```python
from build123d import *

# Parameters (mm, degrees)
ESQUISSE1_W        = 90
ESQUISSE1_H        = 10
BOSS_EXTRU_1_DEPTH = 10
CHANFREIN1_SIZE    = 20


with BuildPart() as part:
    # Esquisse1 → Boss.-Extru.1 (new body)
    with BuildSketch(Plane.XY):
        Polygon((0, 220), (536, 220), (536, 0), (436, 0), (200, 0), (180, 0), (180, 60), (80, 60), (80, 0), (0, 0), align=None)
        with Locations((118, 175)):
            Rectangle(ESQUISSE1_W, ESQUISSE1_H, mode=Mode.SUBTRACT)
        with Locations((268, 175)):
            Rectangle(ESQUISSE1_W, ESQUISSE1_H, mode=Mode.SUBTRACT)
        with Locations((418, 175)):
            Rectangle(ESQUISSE1_W, ESQUISSE1_H, mode=Mode.SUBTRACT)
    extrude(amount=BOSS_EXTRU_1_DEPTH)

    # Chanfrein1
    chanfrein1_edges = [part.edges().sort_by_distance(p)[0] for p in [
        (180, 0, 5),
        (80, 0, 5),
    ]]
    chamfer(chanfrein1_edges, length=CHANFREIN1_SIZE)


solid = part.part
```
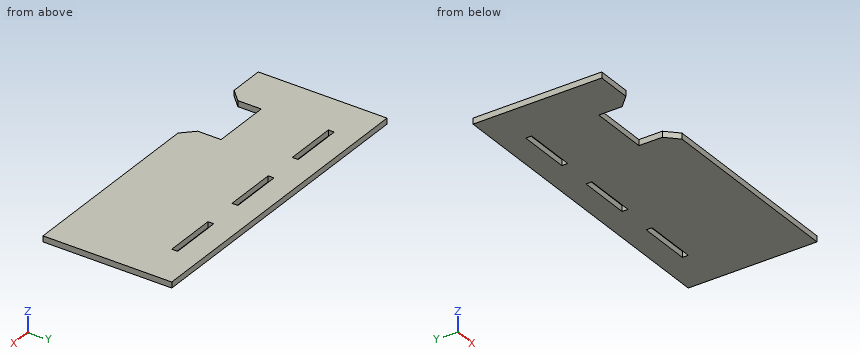
Could you check a few things on this model? Use its own coordinates, in mm. Coordinates: 2 decimals unless noted, no trailing zeros. Order: outer loops, then holes, each group sorted by start corner. A loop starts at its lowest first (then second) coordinate and runs counter-clockwise, first axis right, second up. Notation, with made-up numbers: M 65.5,84 L 120.5,84 A15 ccw 120.5,95 Z; hole C -32.75,3 d11. An arc over 180 degrees is marked long. Use one line per item in the form item = value. Start each with the question number.
1. Suppose I cut it at A-A on y = 39. Write out the boundary of the cut face in (x, z).
2. Suppose I cut it at C-C on x = 302. Write out the boundary of the cut face in (y, z).
3. Suppose I cut it at B-B on z = 6. Write out the boundary of the cut face in (x, y), then the cut area to 3 significant figures.
4. For pin 1 (2 mm diameter, centred on x = 237.5, y = 153, fed in from -Z); pin 2 (2 mm diameter, centred on x = 135, z = 3, fed in from -Y), each with a flat end and sliding along its axis, tell me the tip position at first contact or that it passes through.
5. Please list where these lines run through material, in increasing order: line 1 (Y direction, x = 377.5, z = 5.5); line 2 (X direction, y = 32, z = 7.5); line 3 (Y direction, x = 82, z = 2.25).
6. Suppose I cut it at D-D on x = 185. Write out the boundary of the cut face in (y, z), then the cut area to 3 significant figures.
Geometry says:
q1.outline = M 0,0 L 80,0 L 80,10 L 0,10 Z; M 180,0 L 536,0 L 536,10 L 180,10 Z
q2.outline = M 0,0 L 170,0 L 170,10 L 0,10 Z; M 180,0 L 220,0 L 220,10 L 180,10 Z
q3.outline = M 0,0 L 60,0 L 80,20 L 80,60 L 180,60 L 180,20 L 200,0 L 536,0 L 536,220 L 0,220 Z; hole M 73,170 L 163,170 L 163,180 L 73,180 Z; hole M 223,170 L 313,170 L 313,180 L 223,180 Z; hole M 373,170 L 463,170 L 463,180 L 373,180 Z
q3.area = 109,000 mm^2
q4.pin_1 = 0
q4.pin_2 = 60
q5.line_1 = 0 to 170, 180 to 220
q5.line_2 = 0 to 80, 180 to 536
q5.line_3 = 60 to 170, 180 to 220
q6.outline = M 15,0 L 220,0 L 220,10 L 15,10 Z
q6.area = 2,050 mm^2
